Autodesk Inventor part; units mm, degrees
ref_plane "Work Plane2" through (0, 4, 0) normal (0, 1, 0) x (-1, 0, 0)
ref_plane "YZ Plane" through (0, 0, 0) normal (1, 0, 0) x (0, 1, 0)
ref_plane "XY Plane" through (0, 0, 0) normal (0, 0, 1) x (1, 0, 0)
sketch "Sketch1" plane through (0, 0, 0) normal (0, 1, 0) x (-1, 0, 0)
  line L0 (208, 0) -> (-208, 0)
  line L1 (-228, -20) -> (-228, -52)
  line L2 (-228, -52) -> (-215.25, -52)
  line L3 (-215.25, -52) -> (-215.25, -60)
  line L4 (-215.25, -60) -> (-200.25, -60)
  line L5 (-200.25, -60) -> (-200.25, -52)
  line L6 (-200.25, -52) -> (-176.75, -52)
  line L7 (-176.75, -52) -> (-176.75, -60)
  line L8 (-176.75, -60) -> (-88, -60)
  line L9 (-88, -60) -> (-88, -80)
  line L10 (-88, -80) -> (88, -80)
  line L11 (88, -80) -> (88, -60)
  line L12 (88, -60) -> (176.75, -60)
  line L13 (176.75, -60) -> (176.75, -52)
  line L14 (176.75, -52) -> (200.25, -52)
  line L15 (200.25, -52) -> (200.25, -60)
  line L16 (200.25, -60) -> (215.25, -60)
  line L17 (215.25, -60) -> (215.25, -52)
  line L18 (215.25, -52) -> (228, -52)
  line L19 (228, -52) -> (228, -20)
  line L20 (0, -80) -> (0, 0) construction
  arc A0 (228, -20) -> (208, 0) centre (208, -20) ccw
  arc A1 (-208, 0) -> (-228, -20) centre (-208, -20) ccw
  line L21 (75, -19) -> (-23, -19)
  line L22 (-23, -19) -> (-23, -60)
  line L23 (-23, -60) -> (75, -60)
  line L24 (75, -60) -> (75, -19)
  line L25 (155.25, -4) -> (147.05, -4)
  line L26 (147.05, -4) -> (147.05, -12.2)
  line L27 (147.05, -12.2) -> (155.25, -12.2)
  line L28 (155.25, -12.2) -> (155.25, -4)
  line L29 (155.25, -23) -> (147.05, -23)
  line L30 (147.05, -23) -> (147.05, -31.2)
  line L31 (147.05, -31.2) -> (155.25, -31.2)
  line L32 (155.25, -31.2) -> (155.25, -23)
  line L33 (155.25, -42) -> (147.05, -42)
  line L34 (147.05, -42) -> (147.05, -50.2)
  line L35 (147.05, -50.2) -> (155.25, -50.2)
  line L36 (155.25, -50.2) -> (155.25, -42)
  line L37 (151.15, -42) -> (151.15, -31.2) construction
  line L38 (151.15, -23) -> (151.15, -12.2) construction
  line L39 (-155.25, -4) -> (-147.05, -4)
  line L40 (-147.05, -4) -> (-147.05, -12.2)
  line L41 (-147.05, -12.2) -> (-155.25, -12.2)
  line L42 (-155.25, -12.2) -> (-155.25, -4)
  line L43 (-155.25, -23) -> (-147.05, -23)
  line L44 (-147.05, -23) -> (-147.05, -31.2)
  line L45 (-147.05, -31.2) -> (-155.25, -31.2)
  line L46 (-155.25, -31.2) -> (-155.25, -23)
  line L47 (-155.25, -42) -> (-147.05, -42)
  line L48 (-147.05, -42) -> (-147.05, -50.2)
  line L49 (-147.05, -50.2) -> (-155.25, -50.2)
  line L50 (-155.25, -50.2) -> (-155.25, -42)
  line L51 (-151.15, -42) -> (-151.15, -31.2) construction
  line L52 (-151.15, -23) -> (-151.15, -12.2) construction
  line L53 (79, -69.5) -> (-74, -69.5) construction
  line L54 (-74, -69.5) -> (-74, -18.5) construction
  line L55 (-74, -18.5) -> (79, -18.5) construction
  line L56 (79, -18.5) -> (79, -69.5) construction
  line L57 (-35.5, -40) -> (-69.5, -40) construction
  line L58 (-52.5, -57) -> (-52.5, -23) construction
  line L59 (188, -52) -> (188, -48)
  line L60 (188, -48) -> (189.25, -48)
  line L61 (189.25, -48) -> (189.25, -45)
  line L62 (189.25, -45) -> (188, -45)
  line L63 (188, -45) -> (188, -40)
  line L64 (188, -40) -> (184.5, -40)
  line L65 (184.5, -40) -> (184.5, -45)
  line L66 (184.5, -45) -> (183.25, -45)
  line L67 (183.25, -45) -> (183.25, -48)
  line L68 (183.25, -48) -> (184.5, -48)
  line L69 (184.5, -48) -> (184.5, -52)
  line L70 (-184.5, -52) -> (-184.5, -48)
  line L71 (-184.5, -48) -> (-183.25, -48)
  line L72 (-183.25, -48) -> (-183.25, -45)
  line L73 (-183.25, -45) -> (-184.5, -45)
  line L74 (-184.5, -45) -> (-184.5, -40)
  line L75 (-184.5, -40) -> (-188, -40)
  line L76 (-188, -40) -> (-188, -45)
  line L77 (-188, -45) -> (-189.25, -45)
  line L78 (-189.25, -45) -> (-189.25, -48)
  line L79 (-189.25, -48) -> (-188, -48)
  line L80 (-188, -48) -> (-188, -52)
  point P0 (228, 0)
  point P1 (-228, 0)
  point P2 (151.15, -36.6)
  point P3 (151.15, -17.6)
  point P4 (-151.15, -36.6)
  point P5 (-151.15, -17.6)
  point P6 (-52.5, -40)
  point P7 (-52.5, -40)
  dimension "d0" = 456
  dimension "d1" = 80
  dimension "d2" = 60
  dimension "d3" = 8
  dimension "d4" = 140
  dimension "d5" = 23.5
  dimension "d6" = 15
  dimension "d7" = 12.75
  dimension "d8" = 20
  dimension "d9" = 19
  dimension "d10" = 41
  dimension "d11" = 98
  dimension "d12" = 153
  dimension "d13" = 8.2
  dimension "d14" = 8.2
  dimension "d15" = 72.75
  dimension "d16" = 4
  dimension "d17" = 23
  dimension "d18" = 42
  dimension "d19" = 18.5
  dimension "d20" = 51
  dimension "d21" = 153
  dimension "d22" = 149
  dimension "d23" = 40
  dimension "d24" = 29.5
  dimension "d25" = 34
  dimension "d26" = 34
  dimension "d27" = 4
  dimension "d28" = 3
  dimension "d29" = 5
  dimension "d30" = 6
  dimension "d31" = 3.5
  dimension "d32" = 40
  dimension "d34" = 3.5
  dimension "d35" = 6
  dimension "d36" = 40
extrude "Extrusion1" add sketch "Sketch1" along normal blind 8 contours A0 L19 L18 L17 L16 L15 L14 L59 L60 L61 L62 L63 L64 L65 L66 L67 L68 L69 L13 L12 L11 L10 L9 L8 L7 L6 L70 L71 L72 L73 L74 L75 L76 L77 L78 L79 L80 L5 L4 L3 L2 L1 A1 L0
fillet "Fillet1" radius 10 4 edges at (-88, 4, -60) (-88, 4, -80) (88, 4, -80) (88, 4, -60)
hole "Hole1" at (-151.15, 0, -36.6) at (-151.15, 0, -17.6) at (151.15, 0, -17.6) at (151.15, 0, -36.6) at (-79, 0, -69.5) at (-79, 0, -18.5) at (74, 0, -18.5) at (74, 0, -69.5) direction (0, 1, 0) diameter 3.5 end through all
hole "Hole2" at (35.5, 0, -40) at (52.5, 0, -57) at (52.5, 0, -40) at (69.5, 0, -40) at (52.5, 0, -23) direction (0, 1, 0) diameter 8 end through all
ref_plane "Work Plane2" through (0, 4, 0) normal (0, 1, 0) x (-1, 0, 0)
equation "\"d34\" = d31"
equation "\"d35\" = d30"
equation "\"d36\" = d32"
equation "\"d55\" = 0.5 * THICKNESS"
properties part number "A8-0011"
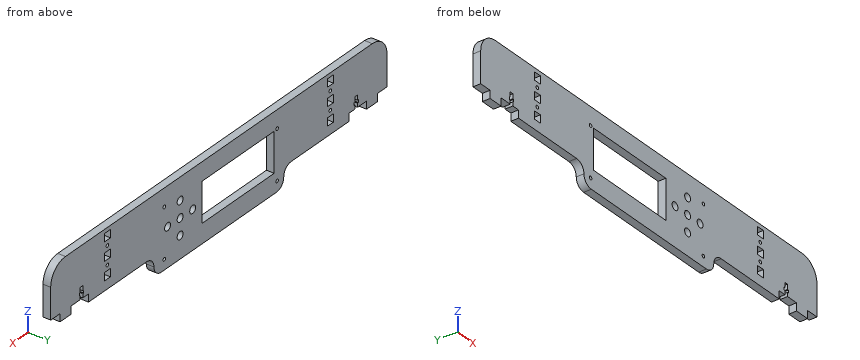
Can you work these out from the model? Positions are in its coordinate system, mm. Give positions to 0.01 mm unless a question says otherwise; leave off trailing zeros. Loops run counter-clockwise (first coordinate to the right, second up) from the corner with the lowest first, then second, coordinate; pieces in that order, holes last. Notation, with made-up numbers: (0.5, 35.5) - (20.5, 35.5) arc R16 cw to (20.5, 58.5) - close; hole circle Ø10 at (0, -38). An arc over 180 degrees is marked (long way). Answer as a JSON object with one key per item and string values.
Q1. Will these pins go through, and if not, where does the flat tip stop? P1, Ø0.6, axis at x = 183.5, y = 2, coming from the -Z side; P2, Ø3, axis at x = -81.5, y = 2.5, coming from the -Z side; P3, Ø4, axis at y = 2.5, z = -7, coming from the +X side; P4, Ø2, axis at x = 56.5, z = -14, coming from the -Y side.
Geometry says:
{"P1": "z = -52", "P2": "z = -79.8", "P3": "x = 224.7", "P4": "y = 0"}
Q2. Imagine slicing it at A-A on x = 1. Write out the boundary of the cut face in (y, z), plus the area to 3 significant figures.
Geometry says:
{"outline": "(0, -80) - (8, -80) - (8, -60) - (0, -60) - close; (0, -19) - (8, -19) - (8, 0) - (0, 0) - close", "area": "312 mm²"}
Q3. Imagine slicing it at C-C on y = 5. Give the number of separate pieces and of enclosed holes in the cut face, plus the area to 3 significant figures.
Geometry says:
{"separate pieces": "1", "enclosed holes": "20", "area": "25,300 mm²"}
Q4. If I drill on L1, parallel to Z at x = 74, y = 2.25; L2, parallel to Z at x = -79, y = 3.75; L3, parallel to Z at x = 52.5, y = 2.5, over which ranges is the centre line in solid material (lowest first)?
Geometry says:
{"L1": "-80 to -71.25, -67.75 to -20.25, -16.75 to 0", "L2": "-79.95 to -71.25, -67.75 to -20.25, -16.75 to 0", "L3": "-80 to -61, -53 to -44, -36 to -27, -19 to 0"}
Q5. Imagine slicing it at B-B on x = 52.5. Write out the boundary of the cut face in (y, z), plus the area to 3 significant figures.
Geometry says:
{"outline": "(0, -80) - (8, -80) - (8, -61) - (0, -61) - close; (0, -53) - (8, -53) - (8, -44) - (0, -44) - close; (0, -36) - (8, -36) - (8, -27) - (0, -27) - close; (0, -19) - (8, -19) - (8, 0) - (0, 0) - close", "area": "448 mm²"}
